Can you work these out from the model? Positions are in its coordinate system, mm. Round coordinates to 2 decimals unless told otherwise and drop trailing zeros. Loops run counter-clockwise (first coordinate to the right, second up) from the corner with the lowest first, then second, coordinate; pieces in that order, holes last. Notation, with made-up numbers: M 13.25,83 L 57.25,83 A15 cw 57.25,103 Z; hole C -28.5,-6 d9. An arc over 180 degrees is marked long. Answer as CSV lines item,"result".
from build123d import *

# Parameters (mm, degrees)
DODANIE_WYCI_GNI_CIE2_DEPTH      = 3
DODANIE_WYCI_GNI_CIE2_DEPTH_BACK = 3
SZKIC1_W                         = 880
SZKIC1_H                         = 74.5
SZKIC1_W_2                       = 736
SZKIC1_H_2                       = 28
SZKIC2_W                         = 40
SZKIC2_H                         = 6
WYTNIJ_WYCI_GNI_CIE1_DEPTH       = 6
SZYK_LINIOWY1_COUNT              = 13
SZYK_LINIOWY1_PITCH              = 91
WYTNIJ_WYCI_GNI_CIE2_DEPTH       = 6
SZKIC4_W                         = 10
SZKIC4_H                         = 15
SZKIC4_H_2                       = 9
SZKIC4_H_3                       = 12
WYTNIJ_WYCI_GNI_CIE3_DEPTH       = 6
WYTNIJ_WYCI_GNI_CIE4_DEPTH       = 6
SZKIC8_R                         = 1.55
SZKIC8_R_2                       = 2.7
WYTNIJ_WYCI_GNI_CIE5_DEPTH       = 6
SZKIC9_R                         = 12.5
WYTNIJ_WYCI_GNI_CIE6_DEPTH       = 6
SZKIC13_W                        = 30
SZKIC13_H                        = 16
WYTNIJ_WYCI_GNI_CIE8_DEPTH       = 6
SZYK_LINIOWY3_COUNT              = 2
SZYK_LINIOWY3_PITCH              = 91
SZYK_LINIOWY3_COUNT_DIR2         = 3
SZYK_LINIOWY3_PITCH_DIR2         = 273
SZKIC15_W                        = 765.002168891
SZKIC15_H                        = 31.530782264
WYTNIJ_WYCI_GNI_CIE9_DEPTH       = 10
SZKIC16_R                        = 1.55
WYTNIJ_WYCI_GNI_CIE10_DEPTH      = 10
SZKIC17_W                        = 24
SZKIC17_H                        = 29.031184719
WYTNIJ_WYCI_GNI_CIE11_DEPTH      = 6
SZKIC20_W                        = 5
SZKIC20_H                        = 10
DODANIE_WYCI_GNI_CIE3_DEPTH      = 6
SZKIC18_W                        = 24.502253475
SZKIC18_H                        = 3.530782264
DODANIE_WYCI_GNI_CIE4_DEPTH      = 6
SZKIC21_W                        = 6.3
SZKIC21_H                        = 26.969217736
DODANIE_WYCI_GNI_CIE5_DEPTH      = 6
SZKIC22_W                        = 10
SZKIC22_H                        = 10
WYTNIJ_WYCI_GNI_CIE12_DEPTH      = 10
SZKIC11_R                        = 3.75
WYTNIJ_WYCI_GNI_CIE7_DEPTH       = 6


with BuildPart() as part:
    # Szkic1 → Dodanie-wyci_gni_cie2 (new, two sides: drawn at the far end of the back side and taken through both)
    with BuildSketch(Plane(origin=(0, -418.87633849, -418.87633849), x_dir=(1, 0, 0), z_dir=(0, 1, 0)).offset(-DODANIE_WYCI_GNI_CIE2_DEPTH_BACK)):
        with Locations((-705.368459045, -446.12633849)):
            Rectangle(SZKIC1_W, SZKIC1_H)
        with Locations((-702.868459045, -438.87633849)):
            Rectangle(SZKIC1_W_2, SZKIC1_H_2, mode=Mode.SUBTRACT)
    extrude(amount=DODANIE_WYCI_GNI_CIE2_DEPTH + DODANIE_WYCI_GNI_CIE2_DEPTH_BACK)

    # Szkic2 → Wytnij-wyci_gni_cie1 (cut)
    with BuildSketch(Plane.XY.offset(64.5)):
        with Locations((-1125.368459045, -418.87633849)):
            Rectangle(SZKIC2_W, SZKIC2_H)
    wytnij_wyci_gni_cie1 = extrude(amount=-WYTNIJ_WYCI_GNI_CIE1_DEPTH, mode=Mode.SUBTRACT)

    # Szyk liniowy1: Wytnij-wyci_gni_cie1 ×13
    with Locations(*[(i * SZYK_LINIOWY1_PITCH, 0, 0) for i in range(1, SZYK_LINIOWY1_COUNT)]):
        add(wytnij_wyci_gni_cie1, mode=Mode.SUBTRACT)

    # Szkic3 → Wytnij-wyci_gni_cie2 (cut)
    with BuildSketch(Plane(origin=(0, -415.87633849, 0), x_dir=(1, 0, 0), z_dir=(0, 1, 0))):
        Polygon((-1032.818459045, -58.5), (-1035.918459045, -58.5), (-1035.918459045, -54.5), (-1037.293459045, -54.5), (-1037.293459045, -52.5), (-1035.918459045, -52.5), (-1035.918459045, -52), (-1032.818459045, -52), (-1032.818459045, -52.5), (-1031.443459045, -52.5), (-1031.443459045, -54.5), (-1032.818459045, -54.5), align=None)
    wytnij_wyci_gni_cie2 = extrude(amount=-WYTNIJ_WYCI_GNI_CIE2_DEPTH, mode=Mode.SUBTRACT)

    # Szkic4 → Wytnij-wyci_gni_cie3 (cut)
    with BuildSketch(Plane(origin=(0, -415.87633849, 0), x_dir=(1, 0, 0), z_dir=(0, 1, 0))):
        with Locations((-1140.368459045, -27)):
            Rectangle(SZKIC4_W, SZKIC4_H)
        with Locations((-1140.368459045, -54)):
            Rectangle(SZKIC4_W, SZKIC4_H_2)
        with Locations((-1140.368459045, 4)):
            Rectangle(SZKIC4_W, SZKIC4_H_3)
    wytnij_wyci_gni_cie3 = extrude(amount=-WYTNIJ_WYCI_GNI_CIE3_DEPTH, mode=Mode.SUBTRACT)

    # Szkic5 → Wytnij-wyci_gni_cie4 (cut)
    with BuildSketch(Plane(origin=(0, -415.87633849, 0), x_dir=(1, 0, 0), z_dir=(0, 1, 0))):
        Polygon((-1135.368459045, 3.55), (-1127.368459045, 3.55), (-1127.368459045, 4.925), (-1125.368459045, 4.925), (-1125.368459045, 3.55), (-1124.868459045, 3.55), (-1124.868459045, 0.45), (-1125.368459045, 0.45), (-1125.368459045, -0.925), (-1127.368459045, -0.925), (-1127.368459045, 0.45), (-1135.368459045, 0.45), align=None)
    wytnij_wyci_gni_cie4 = extrude(amount=-WYTNIJ_WYCI_GNI_CIE4_DEPTH, mode=Mode.SUBTRACT)

    # Lustro1: Wytnij-wyci_gni_cie3, Wytnij-wyci_gni_cie4 across plane
    add(wytnij_wyci_gni_cie3.mirror(Plane.ZY.offset(705.368459045)), mode=Mode.SUBTRACT)
    add(wytnij_wyci_gni_cie4.mirror(Plane.ZY.offset(705.368459045)), mode=Mode.SUBTRACT)

    # Szkic8 → Wytnij-wyci_gni_cie5 (cut)
    with BuildSketch(Plane.XZ.offset(421.87633849)):
        with Locations((-1119.26479978, 39.289778966)):
            Circle(SZKIC8_R)
        with Locations((-1119.26479978, 6.289778966)):
            Circle(SZKIC8_R)
        with Locations((-1118.705640448, 24)):
            Circle(SZKIC8_R_2)
    extrude(amount=-WYTNIJ_WYCI_GNI_CIE5_DEPTH, mode=Mode.SUBTRACT)

    # Szkic9 → Wytnij-wyci_gni_cie6 (cut)
    with BuildSketch(Plane(origin=(0, -415.87633849, 0), x_dir=(1, 0, 0), z_dir=(0, 1, 0))):
        with Locations(Location((-300.706340265, -22.93, 0), (0, 0, 180))):
            Circle(SZKIC9_R)
    extrude(amount=-WYTNIJ_WYCI_GNI_CIE6_DEPTH, mode=Mode.SUBTRACT)

    # Szkic13 → Wytnij-wyci_gni_cie8 (cut)
    with BuildSketch(Plane(origin=(0, -415.87633849, 0), x_dir=(1, 0, 0), z_dir=(0, 1, 0))):
        with Locations((-280.368459045, -56.5)):
            Rectangle(SZKIC13_W, SZKIC13_H)
    extrude(amount=-WYTNIJ_WYCI_GNI_CIE8_DEPTH, mode=Mode.SUBTRACT)

    # Szyk liniowy3: Wytnij-wyci_gni_cie2 2 × 3
    with Locations(*[Vector(1, 0, 0) * (i * SZYK_LINIOWY3_PITCH) + Vector(1, 0, 0) * (j * SZYK_LINIOWY3_PITCH_DIR2) for i in range(SZYK_LINIOWY3_COUNT) for j in range(SZYK_LINIOWY3_COUNT_DIR2) if (i, j) != (0, 0)]):
        add(wytnij_wyci_gni_cie2, mode=Mode.SUBTRACT)

    # Szkic15 → Wytnij-wyci_gni_cie9 (cut)
    with BuildSketch(Plane(origin=(0, -415.87633849, 0), x_dir=(1, 0, 0), z_dir=(0, 1, 0))):
        with Locations((-692.867290015, -48.734608868)):
            Rectangle(SZKIC15_W, SZKIC15_H)
    extrude(amount=-WYTNIJ_WYCI_GNI_CIE9_DEPTH, mode=Mode.SUBTRACT)

    # Szkic16 → Wytnij-wyci_gni_cie10 (cut)
    with BuildSketch(Plane(origin=(0, -415.87633849, 0), x_dir=(1, 0, 0), z_dir=(0, 1, 0))):
        with Locations(Location((-306.36620557, -50.5, 0), (0, 0, 180))):
            Circle(SZKIC16_R)
        with Locations(Location((-1100.368459045, -52.5, 0), (0, 0, 180))):
            Circle(SZKIC16_R)
    extrude(amount=-WYTNIJ_WYCI_GNI_CIE10_DEPTH, mode=Mode.SUBTRACT)

    # Szkic17 → Wytnij-wyci_gni_cie11 (cut)
    with BuildSketch(Plane(origin=(0, -415.87633849, 0), x_dir=(1, 0, 0), z_dir=(0, 1, 0))):
        with Locations((-1082.368459045, -49.984407641)):
            Rectangle(SZKIC17_W, SZKIC17_H)
    extrude(amount=-WYTNIJ_WYCI_GNI_CIE11_DEPTH, mode=Mode.SUBTRACT)

    # Szkic20 → Dodanie-wyci_gni_cie3 (add)
    with BuildSketch(Plane.XZ.offset(421.87633849)):
        with Locations((-292.868459045, 53.5)):
            Rectangle(SZKIC20_W, SZKIC20_H)
    extrude(amount=-DODANIE_WYCI_GNI_CIE3_DEPTH)

    # Szkic18 → Dodanie-wyci_gni_cie4 (add)
    with BuildSketch(Plane.XZ.offset(421.87633849)):
        with Locations((-322.617332308, 34.734608868)):
            Rectangle(SZKIC18_W, SZKIC18_H)
    extrude(amount=-DODANIE_WYCI_GNI_CIE4_DEPTH)

    # Szkic21 → Dodanie-wyci_gni_cie5 (add)
    with BuildSketch(Plane(origin=(0, -415.87633849, 0), x_dir=(1, 0, 0), z_dir=(0, 1, 0))):
        with Locations((-1067.718459045, -19.484608868)):
            Rectangle(SZKIC21_W, SZKIC21_H)
    extrude(amount=-DODANIE_WYCI_GNI_CIE5_DEPTH)

    # Szkic22 → Wytnij-wyci_gni_cie12 (cut)
    with BuildSketch(Plane(origin=(0, -415.87633849, 0), x_dir=(1, 0, 0), z_dir=(0, 1, 0))):
        with Locations((-295.368459045, -53.5)):
            Rectangle(SZKIC22_W, SZKIC22_H)
    extrude(amount=-WYTNIJ_WYCI_GNI_CIE12_DEPTH, mode=Mode.SUBTRACT)

    # Szkic11 → Wytnij-wyci_gni_cie7 (cut)
    with BuildSketch(Plane.XZ.offset(421.87633849)):
        with Locations((-285.206340265, 38.43)):
            Circle(SZKIC11_R)
        with Locations((-316.206340265, 38.43)):
            Circle(SZKIC11_R)
        with Locations((-316.206340265, 7.43)):
            Circle(SZKIC11_R)
        with BuildLine():
            Line((-285.206340265, 3.68), (-290.934328079, 3.68))
            ThreePointArc((-290.934328079, 3.68), (-294.684328079, 7.43), (-290.934328079, 11.18))
            Line((-290.934328079, 11.18), (-285.206340265, 11.18))
            ThreePointArc((-285.206340265, 11.18), (-281.456340265, 7.43), (-285.206340265, 3.68))
        make_face()
    extrude(amount=-WYTNIJ_WYCI_GNI_CIE7_DEPTH, mode=Mode.SUBTRACT)


solid = part.part
Item 1: If we section it at A-A on y = -419.2: State how many separate pieces and enclosed holes the cut face has, then the cut area to 3 significant figures.
Output:
separate pieces,"1"
enclosed holes,"9"
area,"19,000 mm2"
Item 2: If we section it at B-B on x = -821: Write out the boundary of the cut face in (y, z).
Output:
outline,"M -421.88,-10 L -415.88,-10 L -415.88,6 L -421.88,6 Z"
Item 3: We'd pull the mould along Z, two halves only. Please class faces 1 (the face through (-773, -415.876, 2)), 2 (the face through (-312.63, -418.83, 26.68)): released by +Z, released by -Z, zero draft, split by the parting line, or undercut.
Output:
face 1,"zero draft"
face 2,"undercut"
Item 4: Will these pins go through, and if not, where does the flat tip stop? pin 1 (0.7 mm diameter, centred on y = -420, z = 0.5, fed in from +X); pin 2 (3 mm diameter, centred on x = -1116.5, y = -420, fed in from +Z); pin 3 (1.5 mm diameter, centred on y = -416.5, z = 33, fed in from -X).
Output:
pin 1,"stops at x = -275.37"
pin 2,"stops at z = 58.5"
pin 3,"stops at x = -1135.37"
Item 5: If I drill on line 1 along X through (y, z) = (-417.3, 37.5); line 2 along X through (y, z) = (-419.05, 48); line 3 along Z through (x, y) = (-1056, -416.2), over which ranges is the centre line in solid material (lowest first)? Write a range as from..to.
Output:
line 1,"x = -1145.37..-1094.37, -310.37..-288.84, -281.57..-265.37"
line 2,"x = -1145.37..-1094.37, -310.37..-265.37"
line 3,"z = -10..6"
